Input: part model. Units: mm. Frame: model coordinates. A direction names the side the tool comes from. Coordinates: 2 decimals unless noted, no trailing zeros. Put each result on its own line as item: value. Start each with the question number.
1. Pin query (flat end, axial travel): pin 1 (2 mm diameter, centred on x = 9, y = 10, fed in from -Z); pin 2 (4 mm diameter, centred on x = 5.08, y = 5.08, fed in from +Z); pin 3 (1 mm diameter, centred on x = -0.5, z = 4, fed in from +Y). Return the tip coordinate at first contact, or that it passes through.
2. Access query for faces 1 (the flat face through (-1, 12.7, 7)), 2 (the flat face through (0, 6, -3)), 3 (the cylindrical face through (4.39, 1.98, 12.79)), 4 (the cylindrical face through (8.19, 4.94, 1.88)). Directions: +Z, -Z, +X, -X, +Y, -Y. A direction counts if a zero-diameter tool reaches every point of the face in a straight line with its end or side. Return the directions, or none.
3. Pull-direction query (Z, two-part tool) for faces 5 (the flat face through (-1, 3, -5.08)), 6 (the flat face through (6, 0, -3)), 7 (the flat face through (10, 5, 19.05)); classes: released by +Z, released by -Z, zero draft, split by the parting line, or undercut.
4. Line query: line 1 (X direction, y = 5, z = 1); line 2 (Z direction, x = 4.5, y = 35); line 3 (Z direction, x = 3.5, y = 12). Output: solid intervals per line, ascending.
from build123d import *

# Parameters (mm, degrees)
SKETCH1_R                = 3.1115
BOSS_EXTRUDE1_DEPTH      = 3.81
BOSS_EXTRUDE2_DEPTH      = 5.08
BOSS_EXTRUDE2_DEPTH_BACK = 3.81
BOSS_EXTRUDE3_START      = 2.54
SKETCH3_R                = 1.2
BOSS_EXTRUDE3_DEPTH      = 2.54
BOSS_EXTRUDE4_START      = 12.7
SKETCH4_R                = 3.175
BOSS_EXTRUDE4_DEPTH      = 12.7
BOSS_EXTRUDE5_DEPTH      = 12.7
SKETCH7_R                = 3.1115
CUT_EXTRUDE1_DEPTH       = 64.134377028
SKETCH9_R                = 2.000000064
CUT_EXTRUDE2_DEPTH       = 6.99999997
FILLET1_R                = 7.62


with BuildPart() as part:
    # Sketch1 → Boss-Extrude1 (new body)
    with BuildSketch(Plane.XY):
        with BuildLine():
            Line((0, 0), (12.7, 0))
            add(Edge.make_bspline(
                [(0, 12.7), (11.620302725, 11.620302725), (12.7, 0)],
                knots=[0, 0, 0, 1, 1, 1], degree=2))
            Line((0, 12.7), (0, 0))
        make_face()
        with Locations(Location((5.08, 5.08, 0), (0, 0, 180))):
            Circle(SKETCH1_R, mode=Mode.SUBTRACT)
    extrude(amount=BOSS_EXTRUDE1_DEPTH)

    # Sketch2 → Boss-Extrude2 (add, two sides: drawn at the far end of the back side and taken through both)
    with BuildSketch(Plane(origin=(0, 0, 0), x_dir=(-1, 0, 0), z_dir=(0, 0, -1)).offset(-BOSS_EXTRUDE2_DEPTH_BACK)):
        with BuildLine():
            Line((0, 12.7), (1.27, 12.7))
            ThreePointArc((1.27, 12.7), (2.168025612, 12.328025612), (2.54, 11.43))
            Line((2.54, 11.43), (2.54, -1.27))
            ThreePointArc((2.54, -1.27), (2.168025612, -2.168025612), (1.27, -2.54))
            Line((1.27, -2.54), (-11.43, -2.54))
            ThreePointArc((-11.43, -2.54), (-12.328025612, -2.168025612), (-12.7, -1.27))
            Line((-12.7, -1.27), (-12.7, 0))
            Line((-12.7, 0), (0, 0))
            Line((0, 0), (0, 12.7))
        make_face()
    extrude(amount=BOSS_EXTRUDE2_DEPTH + BOSS_EXTRUDE2_DEPTH_BACK)

    # Sketch3 → Boss-Extrude3 (add)
    with BuildSketch(Plane.XY.offset(3.81).offset(BOSS_EXTRUDE3_START)):
        with BuildLine():
            Line((-2.54, 11.43), (-2.54, -1.27))
            ThreePointArc((-2.54, -1.27), (-2.168025612, -2.168025612), (-1.27, -2.54))
            Line((-1.27, -2.54), (11.43, -2.54))
            ThreePointArc((11.43, -2.54), (12.328025612, -2.168025612), (12.7, -1.27))
            Line((12.7, -1.27), (12.7, 0))
            add(Edge.make_bspline(
                [(0, 12.7), (11.620302725, 11.620302725), (12.7, 0)],
                knots=[0, 0, 0, 1, 1, 1], degree=2))
            Line((0, 12.7), (-1.27, 12.7))
            ThreePointArc((-1.27, 12.7), (-2.168025612, 12.328025612), (-2.54, 11.43))
        make_face()
        with Locations((5.08, 5.08)):
            Circle(SKETCH3_R, mode=Mode.SUBTRACT)
    extrude(amount=-BOSS_EXTRUDE3_DEPTH)

    # Sketch4 → Boss-Extrude4 (add)
    with BuildSketch(Plane.XY.offset(6.35).offset(BOSS_EXTRUDE4_START)):
        with BuildLine():
            Line((-2.54, 11.43), (-2.54, -1.27))
            ThreePointArc((-2.54, -1.27), (-2.168025612, -2.168025612), (-1.27, -2.54))
            Line((-1.27, -2.54), (11.43, -2.54))
            ThreePointArc((11.43, -2.54), (12.328025612, -2.168025612), (12.7, -1.27))
            Line((12.7, -1.27), (12.7, 0))
            add(Edge.make_bspline(
                [(0, 12.7), (11.620302725, 11.620302725), (12.7, 0)],
                knots=[0, 0, 0, 1, 1, 1], degree=2))
            Line((0, 12.7), (-1.27, 12.7))
            ThreePointArc((-1.27, 12.7), (-2.168025612, 12.328025612), (-2.54, 11.43))
        make_face()
        with Locations((5.08, 5.08)):
            Circle(SKETCH4_R, mode=Mode.SUBTRACT)
    extrude(amount=-BOSS_EXTRUDE4_DEPTH)

    # Sketch8 → Boss-Extrude5 (add)
    with BuildSketch(Plane.ZY.offset(2.54)):
        Polygon((19.05, 11.43), (19.05, -1.27), (64.010676082, 34.724533506), (57.814573212, 42.464069123), align=None)
    extrude(amount=-BOSS_EXTRUDE5_DEPTH)

    # Sketch7 → Cut-Extrude1 (cut, through all)
    with BuildSketch(Plane.XY.offset(19.05)):
        with Locations(Location((5.08, 5.08, 0), (0, 0, 180))):
            Circle(SKETCH7_R)
    extrude(amount=CUT_EXTRUDE1_DEPTH, mode=Mode.SUBTRACT)

    # Sketch9 → Cut-Extrude2 (cut)
    with BuildSketch(Plane(origin=(0, 44.792641372, 55.95036922), x_dir=(1, 0, 0), z_dir=(0, 0.624970196645459, 0.7806486106469008))):
        with Locations(Location((3.81, -7.939987304, 0), (0, 0, 270))):
            Circle(SKETCH9_R)
    extrude(amount=-CUT_EXTRUDE2_DEPTH, mode=Mode.SUBTRACT)

    # Fillet1
    # the kernel refuses this fillet: 7.62 mm, written as the material it takes off along each edge
    with BuildSketch(Plane(origin=(10.16, 54.369751369, 72.685929245), x_dir=(0, -0.7806486106469015, 0.6249701966454579), z_dir=(0, -0.6249701966454579, -0.7806486106469015))) as fillet1_piece_1_section:
        with BuildLine():
            CenterArc((FILLET1_R, FILLET1_R), FILLET1_R, 180, 90)
            Line((0, FILLET1_R), (0, 0))
            Line((0, 0), (FILLET1_R, 0))
        make_face()
    fillet1_piece_1 = extrude(amount=87.756878503, mode=Mode.PRIVATE)
    fillet1_piece_1 = split(fillet1_piece_1, bisect_by=Plane(origin=(8.453079593, 31.089805897, 19.05), z_dir=(0, 0, 1)), keep=Keep.TOP, mode=Mode.PRIVATE)
    add(fillet1_piece_1, mode=Mode.SUBTRACT)


solid = part.part
Report:
1. pin 1: stops at z = 0
1. pin 2: stops at z = 6.35
1. pin 3: stops at y = 12.7
2. face 1: -Z, +X, -X, +Y
2. face 2: -Z, +X, +Y
2. face 3: none
2. face 4: -Z
3. face 5: released by -Z
3. face 6: zero draft
3. face 7: undercut
4. line 1: x = -2.54 to 1.97, 8.19 to 11.56
4. line 2: z = 48.9 to 54.82, 59.43 to 63.79
4. line 3: z = 0 to 19.05, 19.86 to 35.63
